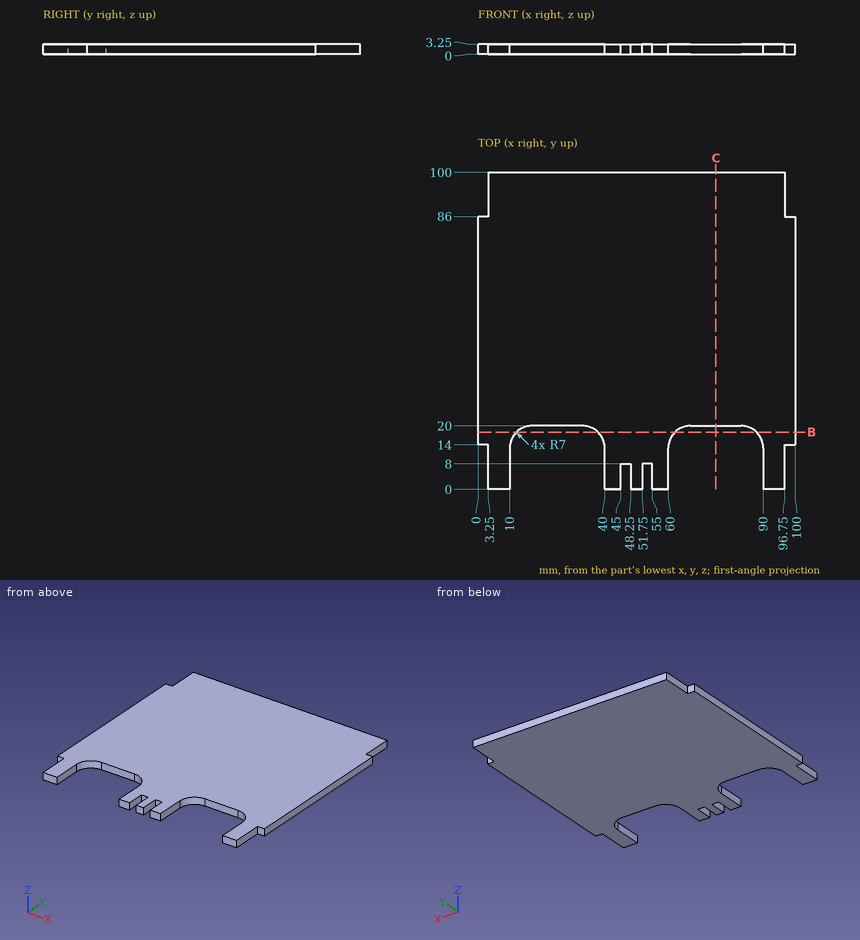
Geometry check sheet. Reference: drawing and pictorial views, mm from the part's lowest x, y, z. Round coordinates to 2 decimals unless told otherwise and drop trailing zeros. Write each loop counter-clockwise with the first axis right and the second up, starting at its lowest first coordinate (ties: lowest second). Pieces come first, ordered by that corner, then holes.
Item 1: Material ranges on line 1 along X through (y, z) = (10.5, 0.6); line 2 along X through (y, z) = (17.5, 3.1); line 3 along X through (y, z) = (90.5, 1.1), recorded low to high.
Determined:
line 1: x = 3.25 to 10, 40 to 60, 90 to 96.75
line 2: x = 0 to 11.64, 38.36 to 61.64, 88.36 to 100
line 3: x = 3.25 to 96.75
Item 2: Section check B-B (y = 18). Record the boundary of the cut face in (x, z), plus the area to 3 significant figures.
Determined:
outline: (0, 0) - (12.1, 0) - (12.1, 3.25) - (0, 3.25) - close; (37.9, 0) - (62.1, 0) - (62.1, 3.25) - (37.9, 3.25) - close; (87.9, 0) - (100, 0) - (100, 3.25) - (87.9, 3.25) - close
area: 157 mm2
Item 3: Section check C-C (x = 75). Record the boundary of the cut face in (y, z).
Determined:
outline: (20, 0) - (100, 0) - (100, 3.25) - (20, 3.25) - close
Item 4: Go/stop test with flat-tipped pins: pin 1 Ø1.6 at (x, z) = (99, 2) entering from -Y; pin 2 Ø1.6 at (y, z) = (5, 2) entering from -X; pin 3 Ø1 at (y, z) = (10, 1.5) entering from +X. Record where each tip stops, or that it passes through.
Determined:
pin 1: stops at y = 14
pin 2: stops at x = 3.25
pin 3: stops at x = 96.75
